Part model, mm, in its own coordinate system. A direction names the side the tool comes from. Round coordinates to 2 decimals unless told otherwise and drop trailing zeros. Write each loop counter-clockwise with the first axis right and the second up, starting at its lowest first coordinate (ties: lowest second). Pieces come first, ordered by that corner, then holes. Notation, with made-up numbers: (-12.75, 30) -> (34.25, 30) arc R11 ccw to (34.25, 50) -> close; hole circle Ø8 at (15.5, -31). An arc over 180 degrees is marked (long way). Use CSV: the item, a comma, the result in double quotes. Start each with the question number.
(1) Two-plate mould, pull along Z, no slides. Class faces 4 (the flat face through (-175, 5, -85)), 5 (the flat face through (-195, 0, -1)), 6 (the cylindrical face through (-147.172, 4.93, 70.01)), 7 (the cylindrical face through (-204.29, 4.93, -75.16)): released by +Z, released by -Z, zero draft, split by the parting line, or undercut.
(2) Saw through at D-D (y = 1.5). Give the cut face in (x, z), plus the area to 3 significant figures.
(3) Drop flat-ended pins along their axis: pin 1 (2.5 mm diameter, centred on y = 2, z = 12, fed in from +X); pin 2 (1 mm diameter, centred on x = -171, z = 55.5, fed in from -Y); pin 3 (3 mm diameter, centred on y = 8.5, z = 2.5, fed in from +X). Give the stop position or say it passes through.
(4) Saw through at B-B (z = -72.5). Give the cut face in (x, y), plus the area to 3 significant figures.
(5) Saw through at A-A (x = -181). Give the cut face in (y, z).
(6) Probe line 1 (Z direction, x = -140, y = 9); line 2 (Z direction, x = -193, y = 1.5); line 3 (X direction, y = 5.75, z = -22). List the from-to ranges inside material, lowest first. Write a range as [from, to].
(7) Which spindle directions (+Z, -Z, +X, -X, +Y, -Y) get a long thin tool onto all of the face, cutting with end or side? Do faces 1 (the flat face through (-133.177, 3, -73)), 2 (the flat face through (-161, 7, -54)), 3 (the flat face through (-188, 5, 0)). Say none if no direction does.
(8) Saw through at C-C (z = 0). Give the cut face in (x, y).
```python
from build123d import *

# Parameters (mm, degrees)
BOSS_EXTRUDE1_DEPTH = 10
CUT_EXTRUDE1_DEPTH  = 5
CHAMFER1_SIZE       = 4
SKETCH3_R           = 6.5
CUT_EXTRUDE2_DEPTH  = 11
SKETCH7_R           = 3
CUT_EXTRUDE3_DEPTH  = 11


with BuildPart() as part:
    # Sketch1 → Boss-Extrude1 (new body)
    with BuildSketch(Plane(origin=(0, 0, 0), x_dir=(1, 0, 0), z_dir=(0, 1, 0))):
        Polygon((-133.17660268, -85), (-133.17660268, -54), (-187.17660268, -54), (-187.17660268, 54), (-133.17660268, 54), (-133.17660268, 85), (-218.17660268, 85), (-218.17660268, -85), align=None)
    extrude(amount=BOSS_EXTRUDE1_DEPTH)

    # Sketch2 → Cut-Extrude1 (cut)
    with BuildSketch(Plane.XZ):
        Polygon((-133.17660268, 60), (-193.17660268, 60), (-193.17660268, -60), (-133.17660268, -60), (-133.17660268, -54), (-187.17660268, -54), (-187.17660268, 54), (-133.17660268, 54), align=None)
    extrude(amount=-CUT_EXTRUDE1_DEPTH, mode=Mode.SUBTRACT)

    # Chamfer1
    chamfer1_edges = [part.edges().sort_by_distance(p)[0] for p in [
        (-133.17660268, 10, 69.5),
        (-133.17660268, 10, -69.5),
    ]]
    chamfer(chamfer1_edges, length=CHAMFER1_SIZE)

    # Sketch3 → Cut-Extrude2 (cut, through all)
    with BuildSketch(Plane.XZ):
        with Locations((-153.17660268, -72.5)):
            Circle(SKETCH3_R)
        with Locations((-153.17660268, 72.5)):
            Circle(SKETCH3_R)
        with Locations((-205.676562711, 0)):
            Circle(SKETCH3_R)
    extrude(amount=-CUT_EXTRUDE2_DEPTH, mode=Mode.SUBTRACT)

    # Sketch7 → Cut-Extrude3 (cut, through all)
    with BuildSketch(Plane.XZ):
        with Locations((-205.67660268, -72.5)):
            Circle(SKETCH7_R)
    extrude(amount=-CUT_EXTRUDE3_DEPTH, mode=Mode.SUBTRACT)


solid = part.part
```
Answers:
1,face 4,"released by -Z"
1,face 5,"zero draft"
1,face 6,"undercut"
1,face 7,"undercut"
2,outline,"(-218.18, -85) -> (-133.18, -85) -> (-133.18, -60) -> (-193.18, -60) -> (-193.18, 60) -> (-133.18, 60) -> (-133.18, 85) -> (-218.18, 85) -> close; hole circle Ø13 at (-205.68, 0); hole circle Ø6 at (-205.68, -72.5); hole circle Ø13 at (-153.18, -72.5); hole circle Ø13 at (-153.18, 72.5)"
2,area,"6,820 mm²"
3,pin 1,"stops at x = -193.18"
3,pin 2,"stops at y = 5"
3,pin 3,"stops at x = -187.18"
4,outline,"(-218.18, 0) -> (-208.68, 0) -> (-208.68, 10) -> (-218.18, 10) -> close; (-202.68, 0) -> (-159.68, 0) -> (-159.68, 10) -> (-202.68, 10) -> close; (-146.68, 0) -> (-133.18, 0) -> (-133.18, 6) -> (-137.18, 10) -> (-146.68, 10) -> close"
4,area,"652 mm²"
5,outline,"(0, -85) -> (10, -85) -> (10, -54) -> (5, -54) -> (5, -60) -> (0, -60) -> close; (0, 60) -> (5, 60) -> (5, 54) -> (10, 54) -> (10, 85) -> (0, 85) -> close"
6,line 1,"z = [-85, -54], [54, 85]"
6,line 2,"z = [-85, -60], [60, 85]"
6,line 3,"x = [-218.18, -187.18]"
7,face 1,"+Z, -Z, +X, +Y, -Y"
7,face 2,"+X, +Y, -Y"
7,face 3,"+X, -Y"
8,outline,"(-218.18, 0) -> (-212.18, 0) -> (-212.18, 10) -> (-218.18, 10) -> close; (-199.18, 0) -> (-193.18, 0) -> (-193.18, 5) -> (-187.18, 5) -> (-187.18, 10) -> (-199.18, 10) -> close"
